```python
from build123d import *

# Parameters (mm, degrees)
F0_R     = 74.956114
F1_DEPTH = 25.4
F2_R     = 47.147248
F3_DEPTH = 25.4
F5_R     = 18.322867
F4_DEPTH = 73.656926


with BuildPart() as f1:
    # F0 (on Front) → F1 (new body)
    with BuildSketch(Plane.XZ):
        Circle(F0_R)
    extrude(amount=F1_DEPTH)

    # F2 (on face) → F3 (intersect)
    with BuildSketch(Plane.XZ.offset(25.4)):
        Circle(F2_R)
    extrude(amount=-F3_DEPTH, mode=Mode.INTERSECT)

    # F5 (on face) → F4 (cut)
    with BuildSketch(Plane.XZ.offset(25.4)):
        Circle(F5_R)
    extrude(amount=-F4_DEPTH, mode=Mode.SUBTRACT)


solid = f1.part
```
Design review of the part built by this model. Coordinates are the model's own, in mm. Coordinates: 2 decimals unless noted, no trailing zeros. Loops run counter-clockwise (first coordinate to the right, second up) from the corner with the lowest first, then second, coordinate; pieces in that order, holes last.
Q1. For pin 1 (5 mm diameter, centred on x = 8, y = -22.5, fed in from -Z); pin 2 (8 mm diameter, centred on y = -19.5, z = 17, fed in from +X); pin 3 (2 mm diameter, centred on y = -16.5, z = -19, fed in from +X), all flat-tipped, find the tip position at first contact; note any pin that passes through.
Reported:
pin 1: stops at z = -46.83
pin 2: stops at x = 45.32
pin 3: stops at x = 43.58
Q2. We need section A-A on z = -5. State the section outline as (x, y) points, and give its area (3 significant figures).
Reported:
outline: (-46.88, -25.4) - (-17.63, -25.4) - (-17.63, 0) - (-46.88, 0) - close; (17.63, -25.4) - (46.88, -25.4) - (46.88, 0) - (17.63, 0) - close
area: 1,490 mm2
Q3. We need section D-D on z = -36. State the section outline as (x, y) points, and give its area (3 significant figures).
Reported:
outline: (-30.44, -25.4) - (30.44, -25.4) - (30.44, 0) - (-30.44, 0) - close
area: 1,550 mm2
Q4. We need section C-C on y = -2. State the section outline as (x, z) points, and give its area (3 significant figures).
Reported:
outline: circle Ø94.29 at (0, 0); hole circle Ø36.65 at (0, 0)
area: 5,930 mm2
Q5. The part is to be moulded in two halves that separate along Z. For faces 1 (the face through (21.756, -12.878, -41.828)), 2 (the face through (-1, -25.4, -20)), 3 (the face through (-18.305, -12.878, 0.806)), say which applies: +Z half, -Z half, draft (parallel to the pull), parting line (faces both ways), or undercut.
Reported:
face 1: parting line
face 2: draft
face 3: undercut
Q6. We need section B-B on x = 0. State the section outline as (y, z) points.
Reported:
outline: (-25.4, -47.15) - (0, -47.15) - (0, -18.32) - (-25.4, -18.32) - close; (-25.4, 18.32) - (0, 18.32) - (0, 47.15) - (-25.4, 47.15) - close
Q7. To check wall thickness, follow line 1 (Z direction, x = 0, y = -17.25); line 2 (Z direction, x = 2.5, y = -7); line 3 (X direction, y = -7.75, z = -15). State the ranges of each line that lie inside material, in increasing order.
Reported:
line 1: z = -47.15 to -18.32, 18.32 to 47.15
line 2: z = -47.08 to -18.15, 18.15 to 47.08
line 3: x = -44.7 to -10.52, 10.52 to 44.7
